from build123d import *

# Parameters (mm, degrees)
F0_R     = 2.5
F1_DEPTH = 2.5


with BuildPart() as f1:
    # F0 (on Front) → F1 (new body)
    with BuildSketch(Plane.XZ):
        with BuildLine():
            Line((10, 4), (0, 4))
            ThreePointArc((0, 4), (-4, 0), (0, -4))
            Line((0, -4), (10, -4))
            ThreePointArc((10, -4), (14, 0), (10, 4))
        make_face()
        Circle(F0_R, mode=Mode.SUBTRACT)
        with BuildLine():
            ThreePointArc((12.5, 0), (10, -2.5), (7.5, 0))
            ThreePointArc((7.5, 0), (10, 2.5), (12.5, 0))
        make_face(mode=Mode.SUBTRACT)
    extrude(amount=F1_DEPTH)


solid = f1.part
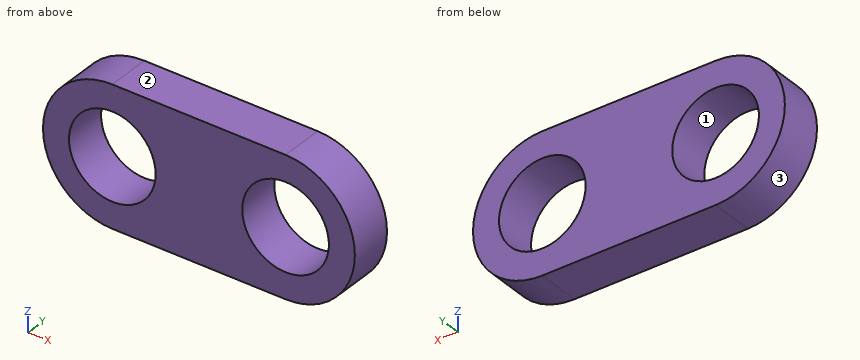
Input: part model. Units: mm. Frame: model coordinates. Face numbers are marked on the shaded views. Coordinates: 2 decimals unless noted, no trailing zeros. Loops run counter-clockwise (first coordinate to the right, second up) from the corner with the lowest first, then second, coordinate; pieces in that order, holes last.
(1) First-contact query: pin 1 Ø4.5 at (x, z) = (10, 0) entering from -Y. Flat tip, straight axial feed; report the tip coordinate or a pass-through.
(2) Section C-C on y = -2.2. Return the cut outline in (x, z).
(3) Pull-direction query (X, two-part tool) for the marked faces 1, 2 and 3; classes: released by +X, released by -X, zero draft, split by the parting line, or undercut.
(4) Section A-A on z = 0. Return the cut outline in (x, y).
(5) Section D-D on z = -1.25. Return the cut outline in (x, y), then the cut area to 3 significant figures.
(6) Section B-B on x = 1.5. Return the cut outline in (y, z).
(7) Material intervals for probe 1 along Z at (x, y) = (0, -1.8); probe 2 along X at (y, z) = (-0.95, -1); probe 3 along X at (y, z) = (-2.2, -1.75), sorted ascending.
Data:
1. pin 1: passes through
2. outline: (0, -4) - (10, -4) arc R4 ccw to (10, 4) - (0, 4) arc R4 ccw to start; hole circle Ø5 at (0, 0); hole circle Ø5 at (10, 0)
3. face 1: undercut
3. face 2: zero draft
3. face 3: released by -X
4. outline: (-4, -2.5) - (-2.5, -2.5) - (-2.5, 0) - (-4, 0) - close; (2.5, -2.5) - (7.5, -2.5) - (7.5, 0) - (2.5, 0) - close; (12.5, -2.5) - (14, -2.5) - (14, 0) - (12.5, 0) - close
5. outline: (-3.8, -2.5) - (-2.17, -2.5) - (-2.17, 0) - (-3.8, 0) - close; (2.17, -2.5) - (7.83, -2.5) - (7.83, 0) - (2.17, 0) - close; (12.17, -2.5) - (13.8, -2.5) - (13.8, 0) - (12.17, 0) - close
5. area: 22.3 mm2
6. outline: (-2.5, -4) - (0, -4) - (0, -2) - (-2.5, -2) - close; (-2.5, 2) - (0, 2) - (0, 4) - (-2.5, 4) - close
7. probe 1: z = -4 to -2.5, 2.5 to 4
7. probe 2: x = -3.87 to -2.29, 2.29 to 7.71, 12.29 to 13.87
7. probe 3: x = -3.6 to -1.79, 1.79 to 8.21, 11.79 to 13.6
